```python
from build123d import *

# Parameters (mm, degrees)
SKETCH1_W           = 30
SKETCH1_H           = 15
SKETCH1_R           = 4.05
BOSS_EXTRUDE1_DEPTH = 15
FILLET1_R           = 8
SKETCH2_W           = 10.1
SKETCH2_H           = 10.1
CUT_EXTRUDE1_DEPTH  = 17
BOSS_EXTRUDE2_DEPTH = 15
CUT_EXTRUDE2_REACH  = 24.191
SKETCH4_R           = 3.2


with BuildPart() as part:
    # Sketch1 → Boss-Extrude1 (new body)
    with BuildSketch(Plane(origin=(0, 0, 0), x_dir=(1, 0, 0), z_dir=(0, 1, 0))):
        Rectangle(SKETCH1_W, SKETCH1_H)
        with Locations(Location((8, 0, 0), (0, 0, 270))):
            Circle(SKETCH1_R, mode=Mode.SUBTRACT)
    extrude(amount=BOSS_EXTRUDE1_DEPTH)

    # Fillet1
    # the kernel refuses this fillet: 8 mm, written as the material it takes off along each edge
    with BuildSketch(Plane(origin=(15, -20, -7.5), x_dir=(-1, 0, 0), z_dir=(0, 1, 0))) as fillet1_piece_1:
        with BuildLine():
            CenterArc((FILLET1_R, FILLET1_R), FILLET1_R, 180, 90)
            Line((0, FILLET1_R), (0, 0))
            Line((0, 0), (FILLET1_R, 0))
        make_face()
    extrude(amount=55, mode=Mode.SUBTRACT)
    with BuildSketch(Plane(origin=(15, -20, 7.5), x_dir=(-1, 0, 0), z_dir=(0, 1, 0))) as fillet1_piece_2:
        with BuildLine():
            CenterArc((FILLET1_R, -FILLET1_R), FILLET1_R, 90, 90)
            Line((0, -FILLET1_R), (0, 0))
            Line((0, 0), (FILLET1_R, 0))
        make_face()
    extrude(amount=55, mode=Mode.SUBTRACT)

    # Sketch2 → Cut-Extrude1 (cut)
    with BuildSketch(Plane.ZY.offset(15)):
        with Locations((0, 7.5)):
            Rectangle(SKETCH2_W, SKETCH2_H)
    extrude(amount=-CUT_EXTRUDE1_DEPTH, mode=Mode.SUBTRACT)

    # Sketch3 → Boss-Extrude2 (add)
    with BuildSketch(Plane.XY.offset(7.5)):
        Polygon((-3, 0), (-9.842158581, -4.145463298), (-15, 0), align=None)
    extrude(amount=-BOSS_EXTRUDE2_DEPTH)

    # Cut-Extrude2: up to this plane
    cut_extrude2_end = Plane(origin=(2, 2.45, 5.05), z_dir=(0, -1, 0))
    # Sketch4 → Cut-Extrude2 (cut, up to the surface)
    with BuildSketch(Plane(origin=(-0.805540592, 1.329558622, 0), x_dir=(0, 0, -1), z_dir=(0.5181829122191232, -0.8552698226198026, 0)), mode=Mode.PRIVATE) as cut_extrude2_sk1:
        with Locations(Location((0, -6.565809468, 0), (0, 0, 90))):
            Circle(SKETCH4_R)
    cut_extrude2_tool1 = split(extrude(cut_extrude2_sk1.sketch, amount=-CUT_EXTRUDE2_REACH, mode=Mode.PRIVATE), bisect_by=cut_extrude2_end, keep=Keep.BOTH, mode=Mode.PRIVATE)
    add(cut_extrude2_tool1.solids().sort_by_distance((-6.421079, -2.072732, 0))[0], mode=Mode.SUBTRACT)


solid = part.part
```
Design review of the part built by this model. Coordinates are the model's own, in mm. A direction names the side the tool comes from. Give positions to 0.01 mm unless a question says otherwise; leave off trailing zeros. Write each loop counter-clockwise with the first axis right and the second up, starting at its lowest first coordinate (ties: lowest second). Pieces come first, ordered by that corner, then holes. Notation, with made-up numbers: (-28, 24.5) - (16, 24.5) arc R10 ccw to (16, 32.5) - close; hole circle Ø3 at (8, -11). An arc over 180 degrees is marked (long way). Return JSON: item names as keys, results as strings. Group by question number.
(1) To check wall thickness, follow probe 1 along X at (y, z) = (8.5, 0); probe 2 along Y at (x, z) = (-2, 1.75); probe 3 along Y at (x, z) = (13.25, 1.5). State the ranges of each line that lie inside material, in increasing order.
(2) We need section B-B, the plane y = 8.75. Give the boundary of the cut face in (x, z), then the cut area to 3 significant figures.
(3) Mouldability with a two-part tool opening along X and no side actions: class faces 1 (the flat face through (-4, 8, 7.5)), 2 (the flat face through (-6.37, -2.04, 3.44)), 3 (the cylindrical face through (9.22, 7.4, 3.86)) as +X half, -X half, draft (parallel to the pull), parting line (faces both ways), or undercut.
(4) Insertion check: pin 1 (5 mm diameter, centred on x = -6.5, z = -1, fed in from -Y); pin 2 (3 mm diameter, centred on y = 7.5, z = 0, fed in from -X); pin 3 (8 mm diameter, centred on x = -11.5, z = 1.5, fed in from -Y); pin 4 (6.5 mm diameter, centred on x = 8, z = 0, fed in from -Y). Each pin has a flat end and moves straight along its axis. Give the tip position at first contact, or say it passes through.
(5) We need section D-D, the plane x = 8. Give the boundary of the cut face in (y, z), then the cut area to 3 significant figures.
(6) We need section C-C, the plane z = 1.75. Give the boundary of the cut face in (x, y).
(7) We need section A-A, the plane x = 0.75. Give the boundary of the cut face in (y, z).
(8) Machinability: for faces 4 (the cylindrical face through (12.4, 7.4, 5.4)), 5 (the flat face through (4, 0, -2)), 6 (the flat face through (-7, 7, 5.05)), which of the approach directions +Z, -Z, +X, -X, +Y, -Y give a long, thin tool a straight path to every point of the face, cutting with its end or side? Answer none if there is none.
Reported:
{
 "1": {"probe 1": "x = 2 to 3.95, 12.05 to 14.98", "probe 2": "y = 0 to 2.45, 12.55 to 15", "probe 3": "y = 0 to 15"},
 "2": {"outline": "(-15, -7.5) - (7, -7.5) arc R8 ccw to (14.98, 0) arc R8 ccw to (7, 7.5) - (-15, 7.5) - (-15, 5.05) - (2, 5.05) - (2, -5.05) - (-15, -5.05) - close; hole circle Ø8.1 at (8, 0)", "area": "199 mm2"},
 "3": {"face 1": "draft", "face 2": "+X half", "face 3": "undercut"},
 "4": {"pin 1": "stops at y = -3.63", "pin 2": "stops at x = 2", "pin 3": "stops at y = -4.15", "pin 4": "passes through"},
 "5": {"outline": "(0, -7.44) - (15, -7.44) - (15, -4.05) - (0, -4.05) - close; (0, 4.05) - (15, 4.05) - (15, 7.44) - (0, 7.44) - close", "area": "102 mm2"},
 "6": {"outline": "(-15, 0) - (-9.84, -4.15) - (-8.71, -3.46) - (-12.29, 2.45) - (-15, 2.45) - close; (-15, 12.55) - (2, 12.55) - (2, 2.45) - (-6.03, 2.45) - (-4.13, -0.68) - (-3, 0) - (4.35, 0) - (4.35, 15) - (-15, 15) - close; (11.65, 0) - (14.68, 0) - (14.68, 15) - (11.65, 15) - close"},
 "7": {"outline": "(0, -7.5) - (15, -7.5) - (15, 7.5) - (0, 7.5) - close; hole (2.45, -5.05) - (12.55, -5.05) - (12.55, 5.05) - (2.45, 5.05) - close"},
 "8": {"face 4": "+Z, +X, +Y, -Y", "face 5": "+Z, -Z, +X, -Y", "face 6": "-X"}
}
